from build123d import *

# Parameters (mm, degrees)
SKETCH1_W           = 160
SKETCH1_H           = 160
BOSS_EXTRUDE1_DEPTH = 9
SKETCH2_W           = 9
SKETCH2_H           = 15
SKETCH2_H_2         = 9
BOSS_EXTRUDE2_DEPTH = 9
SKETCH3_R           = 1.7
SKETCH3_W           = 9
SKETCH3_H           = 15
CUT_EXTRUDE1_DEPTH  = 121.008333044
CUT_EXTRUDE2_DEPTH  = 121.008333044
SKETCH5_R           = 14.825
SKETCH5_R_2         = 11.8
CUT_EXTRUDE3_DEPTH  = 121.008333044


with BuildPart() as part:
    # Sketch1 → Boss-Extrude1 (new body)
    with BuildSketch(Plane(origin=(0, 0, 0), x_dir=(1, 0, 0), z_dir=(0, 1, 0))):
        Rectangle(SKETCH1_W, SKETCH1_H)
    extrude(amount=BOSS_EXTRUDE1_DEPTH)

    # Sketch2 → Boss-Extrude2 (add)
    with BuildSketch(Plane(origin=(0, 9, 0), x_dir=(1, 0, 0), z_dir=(0, 1, 0))):
        with Locations((-84.5, 0)):
            Rectangle(SKETCH2_W, SKETCH2_H)
        with Locations((-84.5, 43.75)):
            Rectangle(SKETCH2_W, SKETCH2_H)
        with Locations((-84.5, -43.75)):
            Rectangle(SKETCH2_W, SKETCH2_H)
        with Locations((-84.5, 75.5)):
            Rectangle(SKETCH2_W, SKETCH2_H_2)
        with Locations((-84.5, -75.5)):
            Rectangle(SKETCH2_W, SKETCH2_H_2)
    extrude(amount=-BOSS_EXTRUDE2_DEPTH)

    # Sketch3 → Cut-Extrude1 (cut, through all)
    with BuildSketch(Plane(origin=(0, 9, 0), x_dir=(1, 0, 0), z_dir=(0, 1, 0))):
        with Locations(Location((70.5, 21.875, 0), (0, 0, 270))):
            Circle(SKETCH3_R)
        with Locations(Location((70.5, -21.875, 0), (0, 0, 270))):
            Circle(SKETCH3_R)
        with Locations((70.5, 43.75)):
            Rectangle(SKETCH3_W, SKETCH3_H)
        with Locations((70.5, 0)):
            Rectangle(SKETCH3_W, SKETCH3_H)
        with Locations((70.5, -43.75)):
            Rectangle(SKETCH3_W, SKETCH3_H)
    extrude(amount=-CUT_EXTRUDE1_DEPTH, mode=Mode.SUBTRACT)

    # Sketch4 → Cut-Extrude2 (cut, through all)
    with BuildSketch(Plane(origin=(0, 9, 0), x_dir=(1, 0, 0), z_dir=(0, 1, 0))):
        Polygon((-80, 23.575), (-76.2, 23.575), (-76.2, 24.625), (-74, 24.625), (-74, 23.575), (-71, 23.575), (-71, 20.175), (-74, 20.175), (-74, 19.125), (-76.2, 19.125), (-76.2, 20.175), (-80, 20.175), align=None)
        Polygon((-80, -23.575), (-80, -20.175), (-76.2, -20.175), (-76.2, -19.125), (-74, -19.125), (-74, -20.175), (-71, -20.175), (-71, -23.575), (-74, -23.575), (-74, -24.625), (-76.2, -24.625), (-76.2, -23.575), align=None)
    extrude(amount=-CUT_EXTRUDE2_DEPTH, mode=Mode.SUBTRACT)

    # Sketch5 → Cut-Extrude3 (cut, through all)
    with BuildSketch(Plane.XZ):
        with Locations(Location((29.011898336, 25.108901907, 0), (0, 0, 270))):
            Circle(SKETCH5_R)
        with Locations(Location((5, -8.301270189, 0), (0, 0, 270))):
            Circle(SKETCH5_R)
        with Locations(Location((-35.940006948, -12.391098093, 0), (0, 0, 270))):
            Circle(SKETCH5_R)
        with Locations(Location((40, -58, 0), (0, 0, 270))):
            Circle(SKETCH5_R_2)
        with Locations(Location((10, -58, 0), (0, 0, 270))):
            Circle(SKETCH5_R_2)
    extrude(amount=-CUT_EXTRUDE3_DEPTH, mode=Mode.SUBTRACT)


solid = part.part
Can you work these out from the model? Positions are in its coordinate system, mm. A direction names the side the tool comes from. Round coordinates to 2 decimals unless told otherwise and drop trailing zeros. Write each loop counter-clockwise with the first axis right and the second up, starting at its lowest first coordinate (ties: lowest second). Pieces come first, ordered by that corner, then holes. Notation, with made-up numbers: M 76,27.5 L 129,27.5 A29 ccw 129,62.5 Z; hole C 52.25,-13.75 d4. An arc over 180 degrees is marked long. Use a Markdown table: item, result.
Item 1: I want a section at D-D (z = -2). List the corners of the cut face in (x, y) for me, and give its area (3 significant figures).
Found:
| item | result |
|---|---|
| outline | M -89,0 L -46.51,0 L -46.51,9 L -89,9 Z; M -25.37,0 L -8.42,0 L -8.42,9 L -25.37,9 Z; M 18.42,0 L 66,0 L 66,9 L 18.42,9 Z; M 75,0 L 80,0 L 80,9 L 75,9 Z |
| area | 1,010 mm2 |
Item 2: We'd pull the mould along X, two halves only. Please class faces 4 (the face through (-89, 5, 76)), 5 (the face through (-85, 5, 71)), 6 (the face through (75, 5, 44)): released by +X, released by -X, zero draft, split by the parting line, or undercut.
Found:
| item | result |
|---|---|
| face 4 | released by -X |
| face 5 | zero draft |
| face 6 | undercut |
Item 3: Which directions (+Z, -Z, +X, -X, +Y, -Y) give clear straight access to the entire face, cutting with the end or side of a thin tool? Please do faces 1 (the face through (-89, 5, -44)), 2 (the face through (-78, 5, -20.175)), 3 (the face through (66, 5, -44)).
Found:
| item | result |
|---|---|
| face 1 | +Z, -Z, -X, +Y, -Y |
| face 2 | -X, +Y, -Y |
| face 3 | +Y, -Y |
Item 4: I want a section at A-A (z = -58). List the corners of the cut face in (x, y) for me.
Found:
| item | result |
|---|---|
| outline | M -80,0 L -1.8,0 L -1.8,9 L -80,9 Z; M 21.8,0 L 28.2,0 L 28.2,9 L 21.8,9 Z; M 51.8,0 L 80,0 L 80,9 L 51.8,9 Z |
Item 5: For pin 1 Ø1 at (y, z) = (4, 28) entering from -X, with a flat end and sliding along its axis, tell me the tip position at first contact or that it passes through.
Found:
| item | result |
|---|---|
| pin 1 | stops at x = -80 |
Item 6: I want a section at C-C (x = -25.5). List the corners of the cut face in (y, z) for me, and give its area (3 significant figures).
Found:
| item | result |
|---|---|
| outline | M 0,-80 L 9,-80 L 9,-22.92 L 0,-22.92 Z; M 0,-1.87 L 9,-1.87 L 9,80 L 0,80 Z |
| area | 1,250 mm2 |
Item 7: If I drill on line 1 along Z through (x, y) = (70.5, 3) (3 decimals); line 2 along Z through (x, y) = (-71.5, 8.25) (3 decimals); line 3 along X through (y, z) = (3, -57.5), over which ranges is the centre line in solid material (lowest first)? Write a range as [from, to].
Found:
| item | result |
|---|---|
| line 1 | z = [-80, -51.25], [-36.25, -23.575], [-20.175, -7.5], [7.5, 20.175], [23.575, 36.25], [51.25, 80] |
| line 2 | z = [-80, -23.575], [-20.175, 20.175], [23.575, 80] |
| line 3 | x = [-80, -1.79], [21.79, 28.21], [51.79, 80] |
Item 8: I want a section at B-B (x = 40). List the corners of the cut face in (y, z) for me.
Found:
| item | result |
|---|---|
| outline | M 0,-80 L 9,-80 L 9,-69.8 L 0,-69.8 Z; M 0,-46.2 L 9,-46.2 L 9,15.16 L 0,15.16 Z; M 0,35.06 L 9,35.06 L 9,80 L 0,80 Z |
